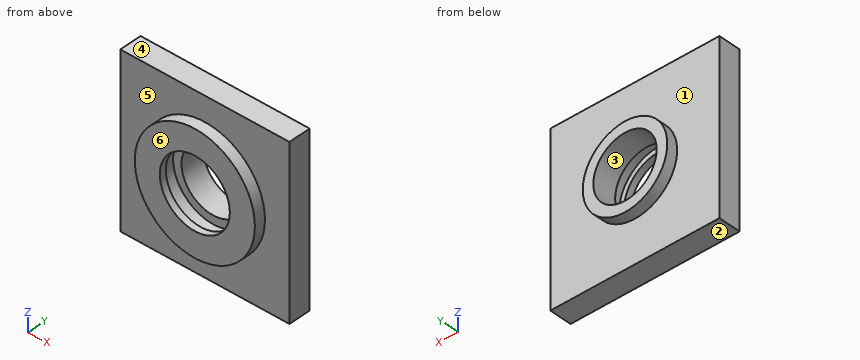
Autodesk Inventor part; units mm, degrees
ref_plane "YZ Plane" through (0, 0, 0) normal (1, 0, 0) x (0, 1, 0)
ref_plane "XZ Plane" through (0, 0, 0) normal (0, 1, 0) x (-1, 0, 0)
ref_plane "XY Plane" through (0, 0, 0) normal (0, 0, 1) x (1, 0, 0)
sketch "Sketch1" plane through (0, 0, 0) normal (0, 1, 0) x (-1, 0, 0)
  line L0 (0, 0) -> (76, 0)
  line L1 (76, 0) -> (76, -76)
  line L2 (76, -76) -> (0, -76)
  line L3 (0, -76) -> (0, 0)
  dimension "d0" = 76
  dimension "d1" = 76
extrude "Extrusion1" add sketch "Sketch1" along normal blind 10
sketch "Sketch2" plane through (0, 10, 0) normal (0, 1, 0) x (1, 0, 0)
  circle A0 centre (-38, 38) radius 19
  point P0 (0, 0)
  dimension "d4" = 38
extrude "Extrusion2" add sketch "Sketch2" along normal blind 4.9
sketch "Sketch8" plane through (0, 0, 0) normal (0, -1, 0) x (1, 0, 0)
  circle A0 centre (-38, -38) radius 27
  point P0 (0, 0)
  dimension "d18" = 54
extrude "Extrusion6" add sketch "Sketch8" along normal blind 5
sketch "Sketch9" plane through (-38, -5, -38) normal (0, -1, 0) x (1, 0, 0)
  circle A0 centre (0, 0) radius 15.75
  point P0 (38, 38)
  dimension "d21" = 31.5
extrude "Extrusion7" cut sketch "Sketch9" against normal blind 3
sketch "Sketch10" plane through (-38, -2, -38) normal (0, -1, 0) x (1, 0, 0)
  circle A0 centre (0, 0) radius 18
  point P0 (38, 38)
  dimension "d24" = 36
extrude "Extrusion8" cut sketch "Sketch10" against normal blind 6.1
sketch "Sketch11" plane through (-38, 14.9, -38) normal (0, 1, 0) x (1, 0, 0)
  circle A0 centre (0, 0) radius 15.75
  circle A1 centre (0, 0) radius 14.25
  point P0 (38, -38)
  dimension "d27" = 28.5
extrude "Extrusion9" cut sketch "Sketch11" against normal blind 10.8 contours A1
Read the model definition and answer for the solid it produces. Units are mm, in the model's axes. Face numbers are marked on the shaded views. A direction names the side the tool comes from. Give positions to 0.01 mm unless a question says otherwise; leave off trailing zeros. Loops run counter-clockwise (first coordinate to the right, second up) from the corner with the lowest first, then second, coordinate; pieces in that order, holes last.
Item 1: Each of these flat-tipped pins is pushed along its axis until it touches: pin 1 Ø5 at (x, z) = (-32.5, -50) entering from -Y; pin 2 Ø3 at (x, z) = (-22.5, -67.5) entering from -Y; pin 3 Ø1.5 at (x, z) = (-65, -62.5) entering from +Y. Where does it stop, or does it pass through?
Item 2: For the marked faces 5 and 6, determine the directions among +Z, -Z, +X, -X, +Y, -Y from which every point of the face is accessible in a straight line to the end or side of a thin tool.
Item 3: The part is cut by section B-B (x = -38). Write down the section's boundary in (y, z), and give its area (3 significant figures).
Item 4: The part is cut by section D-D (x = -68.5). Write down the section's boundary in (y, z).
Item 5: The part is cut by section C-C (y = 5.25). Write down the section's boundary in (x, z).
Item 6: The mould has two halves that part along Z. Classify the marked faces 1, 2, 3 and 4: released by +Z, released by -Z, zero draft, split by the parting line, or undercut.
Item 7: Find the intervals of material crossed by line 1 along Y through (x, z) = (-54.5, -34); line 2 along Z through (x, y) = (-38, 7); line 3 along Z through (x, y) = (-38, -0.5), in increasing order.
Item 8: The part is cut by section A-A (z = -38). Write down the section's boundary in (x, y).
Taken from the geometry:
1. pin 1: stops at y = 4.1
1. pin 2: stops at y = 0
1. pin 3: stops at y = 10
2. face 5: -Y
2. face 6: +Z, -Z, +X, -X, -Y
3. outline: (-5, -65) - (0, -65) - (0, -76) - (10, -76) - (10, -57) - (14.9, -57) - (14.9, -52.25) - (4.1, -52.25) - (4.1, -56) - (-2, -56) - (-2, -53.75) - (-5, -53.75) - close; (-5, -22.25) - (-2, -22.25) - (-2, -20) - (4.1, -20) - (4.1, -23.75) - (14.9, -23.75) - (14.9, -19) - (10, -19) - (10, 0) - (0, 0) - (0, -11) - (-5, -11) - close
3. area: 594 mm2
4. outline: (0, -76) - (10, -76) - (10, 0) - (0, 0) - close
5. outline: (-76, -76) - (0, -76) - (0, 0) - (-76, 0) - close; hole circle Ø28.5 at (-38, -38)
6. face 1: zero draft
6. face 2: released by -Z
6. face 3: undercut
6. face 4: released by +Z
7. line 1: y = -5 to -2, 4.1 to 14.9
7. line 2: z = -76 to -52.25, -23.75 to 0
7. line 3: z = -65 to -56, -20 to -11
8. outline: (-76, 0) - (-65, 0) - (-65, -5) - (-53.75, -5) - (-53.75, -2) - (-56, -2) - (-56, 4.1) - (-52.25, 4.1) - (-52.25, 14.9) - (-57, 14.9) - (-57, 10) - (-76, 10) - close; (-23.75, 4.1) - (-20, 4.1) - (-20, -2) - (-22.25, -2) - (-22.25, -5) - (-11, -5) - (-11, 0) - (0, 0) - (0, 10) - (-19, 10) - (-19, 14.9) - (-23.75, 14.9) - close
